Solid Edge part; units mm, degrees
sketch "Sketch1" plane through (0, 0, 0) normal (1, 0, 0) x (0, 1, 0)
  circle A0 centre (-30.3013, -33.6124) radius 15
  circle A1 centre (-30.3013, -33.6124) radius 30
extrude "Protrusion1" add sketch "Sketch1" along normal mid plane 80
sketch "Sketch2" plane through (0, 0, 0) normal (1, 0, 0) x (0, 1, 0)
  line L0 (-30.3013, 32.3876) -> (-57.023, -19.976)
  arc A0 (-30.3013, -3.6124) -> (-57.023, -19.976) centre (-30.3013, -33.6124) ccw
  line L1 (-30.3013, -3.6124) -> (-30.3013, 32.3876)
extrude "ExtrudedProtrusion_2" add sketch "Sketch2" along normal mid plane 12
sketch "Sketch3" plane through (0, 0, 0) normal (1, 0, 0) x (0, 1, 0)
  line L0 (-30.3013, 32.3876) -> (-10.3013, 32.3876)
  line L1 (-10.3013, 32.3876) -> (-10.3013, 12.3876)
  line L2 (-10.3013, -11.2517) -> (-10.3013, 12.3876)
  arc A0 (-30.3013, -3.6124) -> (-10.3013, -11.2517) centre (-30.3013, -33.6124) cw
  line L3 (-30.3013, -3.6124) -> (-30.3013, 32.3876)
extrude "ExtrudedProtrusion_3" add sketch "Sketch3" along normal mid plane 60
sketch "Sketch4" plane through (0, -20.3013, 32.3876) normal (0, 0, 1) x (0, 1, 0)
  line L0 (-10, 30) -> (-10, -30)
  line L1 (-10, -30) -> (30, -30)
  arc A0 (30, 30) -> (30, -30) centre (30, 0) cw
  line L2 (-10, 30) -> (30, 30)
extrude "ExtrudedProtrusion_5" add sketch "Sketch4" against normal blind 20
sketch "Sketch5" plane through (0, 0, 0) normal (1, 0, 0) x (0, 1, 0)
  line L0 (9.6987, 32.3876) -> (9.6987, 72.3876)
  line L1 (9.6987, 72.3876) -> (29.6987, 72.3876)
  line L2 (29.6987, 72.3876) -> (39.6987, 32.3876)
  line L3 (39.6987, 32.3876) -> (9.6987, 32.3876)
revolve "RevolvedProtrusion1" add sketch "Sketch5" angle 360 about axis through (0, 9.6987, 32.3876) along (0, 0, 1)
sketch "Sketch6" plane through (0, 9.6987, 72.3876) normal (0, 0, 1) x (0, 1, 0)
  circle A0 centre (0, 0) radius 10
extrude "ExtrudedCutout_1" cut sketch "Sketch6" against normal blind 40
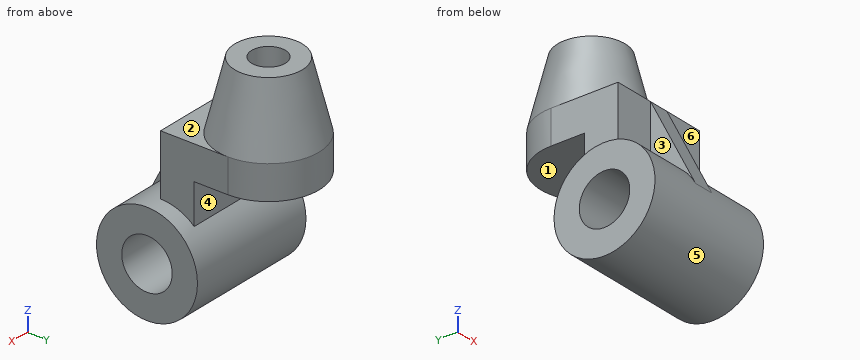
Work out the finished part from the listing and answer in its coordinate system (mm). Face numbers are marked on the shaded views. A direction names the side the tool comes from. Coordinates: 2 decimals unless noted, no trailing zeros. Loops run counter-clockwise (first coordinate to the right, second up) from the corner with the lowest first, then second, coordinate; pieces in that order, holes last. Notation, with made-up numbers: (66, -39) -> (93, -39) arc R21 ccw to (93, -25) -> close; hole circle Ø10 at (42.25, 25.25). An arc over 180 degrees is marked (long way). Answer as CSV lines item,"result".
1) Flat-ended cylindrical pins translate along their axes: pin 1 (3 mm diameter, centred on x = 28.5, z = 14.5, fed in from +Y); pin 2 (15 mm diameter, centred on x = -13.5, y = 17.5, fed in from -Z); pin 3 (1.5 mm diameter, centred on x = -13.5, z = -35, fed in from +Y). Find the tip coordinate at first contact, or state that the pin passes through.
A:
pin 1,"stops at y = 22.78"
pin 2,"stops at z = 12.39"
pin 3,"stops at y = -0.31"
2) The part is cut by section B-B (x = 0). Give the vertices of the cut face in (y, z), and give its area (3 significant figures).
A:
outline,"(-57.02, -19.98) arc R30 ccw (long way) to (-10.3, -11.25) -> (-10.3, 12.39) -> (39.7, 12.39) -> (39.7, 32.39) -> (29.7, 72.39) -> (19.7, 72.39) -> (19.7, 32.39) -> (-0.3, 32.39) -> (-0.3, 72.39) -> (-10.3, 72.39) -> (-20.3, 32.39) -> (-30.3, 32.39) -> close; hole circle Ø30 at (-30.3, -33.61)"
area,"5,480 mm²"
3) The part is cut by section A-A (y = -41.5). Give the vertices of the cut face in (x, z).
A:
outline,"(-40, -61.44) -> (40, -61.44) -> (40, -43.59) -> (-40, -43.59) -> close; (-40, -23.63) -> (40, -23.63) -> (40, -5.78) -> (6, -5.78) -> (6, 10.44) -> (-6, 10.44) -> (-6, -5.78) -> (-40, -5.78) -> close"
4) Straight lines are drawn through the part: probe 1 along Y at (x, z) = (-22.5, -0.5); probe 2 along Z at (x, y) = (-17, 10); probe 3 along X at (y, z) = (-21.5, 4). For each, find the intervals that lie inside material, in ascending order.
A:
probe 1,"y = -30.3 to -10.3"
probe 2,"z = 12.39 to 72.39"
probe 3,"x = -30 to 30"
5) The part is cut by section D-D (z = 47). Give the vertices of the cut face in (x, y), and give its area (3 significant figures).
A:
outline,"circle Ø52.69 at (0, 9.7); hole circle Ø20 at (0, 9.7)"
area,"1,870 mm²"
6) For the marked faces 4, 5 and 6, determine the directions among +Z, -Z, +X, -X, +Y, -Y from which every point of the face is accessible in a straight line to the end or side of a thin tool.
A:
face 4,"+X, -X, +Y"
face 5,"none"
face 6,"+Z, +X, -Y"
7) For a pull along Z with two mould halves and no side action, classify the marked faces 1, 2 and 3 as released by +Z, released by -Z, zero draft, split by the parting line, or undercut.
A:
face 1,"undercut"
face 2,"released by +Z"
face 3,"zero draft"
8) The part is cut by section C-C (z = 29). Give the vertices of the cut face in (x, y), and give its area (3 significant figures).
A:
outline,"(-30, -30.3) -> (-6, -30.3) -> (-6, -32.03) -> (6, -32.03) -> (6, -30.3) -> (30, -30.3) -> (30, 9.7) arc R30 ccw to (-30, 9.7) -> close"
area,"3,830 mm²"
